from build123d import *

# Parameters (mm, degrees)
SKETCH3_W              = 88
SKETCH3_H              = 215
BOSS_EXTRUDE3_DEPTH    = 1.1
CUT_EXTRUDE1_OUTLINE_W = 12
CUT_EXTRUDE1_OUTLINE_H = 13.99905087
CUT_EXTRUDE1_OUTLINE_R = 1.5
CUT_EXTRUDE1_DEPTH     = 1.1
SKETCH5_W              = 13.1
SKETCH5_H              = 5.72
CUT_EXTRUDE3_DEPTH     = 1.1


# Read off the part's stored shape, not the designer's step: Cut-Extrude1
with BuildPart() as part:
    # Sketch3 → Boss-Extrude3 (new body)
    with BuildSketch(Plane.XY):
        with Locations((0.594511969, -70.924817192)):
            Rectangle(SKETCH3_W, SKETCH3_H)
    extrude(amount=BOSS_EXTRUDE3_DEPTH)

    # Cut-Extrude1 outline → Cut-Extrude1 (cut)
    with BuildSketch(Plane.XY):
        with Locations((-37.405488031, 29.575657373)):
            Rectangle(CUT_EXTRUDE1_OUTLINE_W, CUT_EXTRUDE1_OUTLINE_H)
        with Locations((31.594511969, 31.075182808)):
            Circle(CUT_EXTRUDE1_OUTLINE_R)
        with Locations((-38.905488031, -166.424817192)):
            Circle(CUT_EXTRUDE1_OUTLINE_R)
        with Locations((-38.905488031, -70.924817192)):
            Circle(CUT_EXTRUDE1_OUTLINE_R)
        with Locations((-38.905488031, 10.255182808)):
            Circle(CUT_EXTRUDE1_OUTLINE_R)
        with Locations((40.094511969, -70.924817192)):
            Circle(CUT_EXTRUDE1_OUTLINE_R)
        with Locations((40.094511969, -173.424817192)):
            Circle(CUT_EXTRUDE1_OUTLINE_R)
    extrude(amount=CUT_EXTRUDE1_DEPTH, mode=Mode.SUBTRACT)

    # Sketch5 → Cut-Extrude3 (cut)
    with BuildSketch(Plane.XY.offset(1.1)):
        with Locations((22.654511969, -171.524817192)):
            Rectangle(SKETCH5_W, SKETCH5_H)
    extrude(amount=-CUT_EXTRUDE3_DEPTH, mode=Mode.SUBTRACT)


solid = part.part
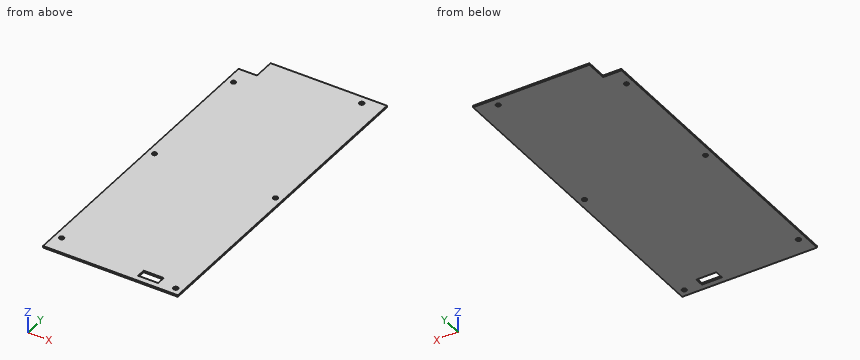
Geometry check sheet. Reference: the model listing, model coordinates, mm. Give positions to 0.01 mm unless a question says otherwise; leave off trailing zeros. Order: outer loops, then holes, each group sorted by start corner. A loop starts at its lowest first (then second) coordinate and runs counter-clockwise, first axis right, second up. Notation, with made-up numbers: M 63,30.5 L 70,30.5 A13 ccw 70,35.5 Z; hole C -30,-5.5 d6. An arc over 180 degrees is marked long. Use a Markdown table: item, result.
Item 1: Section check A-A (x = 22). Record the cut outline in (y, z), and give its area (3 significant figures).
Answers follow:
| item | result |
|---|---|
| outline | M -178.42,0 L -174.38,0 L -174.38,1.1 L -178.42,1.1 Z; M -168.66,0 L 36.58,0 L 36.58,1.1 L -168.66,1.1 Z |
| area | 230 mm2 |
Item 2: Section check B-B (z = 0.6). Record the cut outline in (x, y), and give its area (3 significant figures).
Answers follow:
| item | result |
|---|---|
| outline | M -43.41,-178.42 L 44.59,-178.42 L 44.59,36.58 L -31.41,36.58 L -31.41,22.58 L -43.41,22.58 Z; hole C -38.91,-166.42 d3; hole C -38.91,-70.92 d3; hole C -38.91,10.26 d3; hole M 16.1,-174.38 L 29.2,-174.38 L 29.2,-168.66 L 16.1,-168.66 Z; hole C 31.59,31.08 d3; hole C 40.09,-173.42 d3; hole C 40.09,-70.92 d3 |
| area | 18,600 mm2 |
Item 3: Material ranges on line 1 along Y through (x, z) = (-39, 0.2); line 2 along Y through (x, z) = (-37, 0.1); line 3 along Y through (x, z) = (25, 0.45), recorded low to high.
Answers follow:
| item | result |
|---|---|
| line 1 | y = -178.42 to -167.92, -164.93 to -72.42, -69.43 to 8.76, 11.75 to 22.58 |
| line 2 | y = -178.42 to 22.58 |
| line 3 | y = -178.42 to -174.38, -168.66 to 36.58 |
